Input: part model. Units: mm. Frame: model coordinates. A direction names the side the tool comes from. Coordinates: 2 decimals unless noted, no trailing zeros. Loops run counter-clockwise (first coordinate to the right, second up) from the corner with the lowest first, then second, coordinate; pieces in that order, holes last.
(1) Line query: L1, parallel to Z at x = -2.75, y = 0.9; L2, parallel to Z at x = -1.5, y = 2.5; L3, parallel to Y at x = 0.5, z = -9. Output: solid intervals per line, ascending.
(2) Contact query for flat-ended pins moving along their axis: P1, Ø4, axis at x = -2.75, z = 14, coming from the +Y side; P2, Ø1.2, axis at x = 5, y = 9, coming from the -Z side; P3, Ø2, axis at x = -3.5, z = -14.5, coming from the -Y side. Output: stop coordinate, or through.
(3) Section C-C, the plane x = -2.75. Return loops of the section in (y, z), then the cut area to 3 significant figures.
(4) Mould query, pull axis Y, two halves, no side actions, for faces 1 (the face through (1, 2, -17)), 2 (the face through (0.1, 3.1, -9.8)), 3 (the face through (0, 5, -11)). Classes: released by +Y, released by -Y, zero draft, split by the parting line, or undercut.
(5) Section B-B, the plane z = 14. Return loops of the section in (x, y).
(6) Section D-D, the plane z = 9. Return loops of the section in (x, y), then the cut area to 3 significant figures.
(7) Set-up query: faces 4 (the face through (0, 5, 11)), 5 (the face through (-1, 2, -5)), 6 (the face through (4, 8, -5)). Return all of +Z, -Z, +X, -X, +Y, -Y with unobstructed straight access to the full face (end or side cutting, diameter ignored); none if empty.
(8) Section A-A, the plane x = 0.5. Return loops of the section in (y, z), then the cut area to 3 significant figures.
Autodesk Inventor part; units mm, degrees
ref_plane "Work Plane4" through (0, 2, 0) normal (0, -1, 0) x (1, 0, 0)
ref_plane "YZ Plane" through (0, 0, 0) normal (1, 0, 0) x (0, 1, 0)
ref_plane "XZ Plane" through (0, 0, 0) normal (0, 1, 0) x (-1, 0, 0)
sketch "Sketch1" plane through (0, 0, 0) normal (0, 1, 0) x (-1, 0, 0)
  line L0 (3.75, 17) -> (-5.75, 17)
  line L1 (-5.75, 17) -> (-5.75, -17)
  line L2 (-5.75, -17) -> (3.75, -17)
  line L3 (5.75, 17) -> (-5.75, -17) construction
  line L4 (-5.75, 17) -> (5.75, -17) construction
  arc A0 (5.75, 15) -> (3.75, 17) centre (3.75, 15) ccw
  arc A1 (3.75, -17) -> (5.75, -15) centre (3.75, -15) ccw
  line L5 (-3.25, 0) -> (-3.25, 5)
  line L6 (-3.25, 0) -> (-3.25, -5)
  line L7 (-3.25, -5) -> (5.75, -5)
  line L8 (-3.25, 5) -> (5.75, 5)
  line L9 (5.75, 5) -> (5.75, 15)
  line L10 (5.75, -5) -> (5.75, -15)
  arc A2 (-0.5666, 5) -> (-0.5666, -5) centre (2.75, 0) ccw
  line L11 (-3.25, 5) -> (-5.75, 5)
  line L12 (-3.25, -5) -> (-5.75, -5)
  point P0 (2.75, 14)
  point P1 (2.75, -14)
  dimension "d0" = 11.5
  dimension "d1" = 34
  dimension "d2" = 2
  dimension "d29" = 5
  dimension "d30" = 5
  dimension "d31" = 9
  dimension "d32" = 9
  dimension "d48" = 8.5
extrude "Extrusion1" add sketch "Sketch1" along normal blind 5 contours A0 L9 L8 L11 L1 L0 | L11 L5 L6 L12 L1 | L12 L7 L10 A1 L2 L1
hole "Hole1" at (-2.75, 0, 14) at (-2.75, 0, -14) direction (0, 1, 0) diameter 3.5 depth 8
sketch "Sketch5" plane through (-5.75, 0, 5) normal (-1, 0, 0) x (0, 0, 1)
  point P0 (-5, 0)
  point P1 (4, 2.5)
  point P2 (-14, 2.5)
hole "Hole3" at (-5.75, 2.5, 9) at (-5.75, 2.5, -9) direction (1, 0, 0) diameter 2 depth 12
extrude "Extrusion4" add sketch "Sketch1" along normal blind 10.5 contours L11 L5 L6 L12 L1
ref_plane "Work Plane4" through (0, 2, 0) normal (0, -1, 0) x (1, 0, 0)
sketch "Sketch9" plane through (0, 2, 0) normal (0, -1, 0) x (1, 0, 0)
  circle A0 centre (-2.75, -14) radius 1.75
  circle A1 centre (-2.75, 14) radius 1.75
  circle A2 centre (-2.75, 14) radius 2
  circle A3 centre (-2.75, -14) radius 2
  point P0 (0, 0)
  dimension "d61" = 4
  dimension "d62" = 4
extrude "Extrusion7" cut sketch "Sketch9" along normal blind 10
properties part number "togh" material "ABS Plastic"
Report:
1. L1: z = -17 to -16, -12 to -5, 5 to 12, 16 to 17
1. L2: z = -17 to -15.22, -12.78 to -10, -8 to -5, 5 to 8, 10 to 12.78, 15.22 to 17
1. L3: y = 0 to 1.5, 3.5 to 5
2. P1: stops at y = 5
2. P2: stops at z = -5
2. P3: stops at y = 2
3. outline: (0, -17) - (5, -17) - (5, -15.75) - (2, -15.75) - (2, -16) - (0, -16) - close; (0, -12) - (2, -12) - (2, -12.25) - (5, -12.25) - (5, -5) - (0, -5) - close; (0, 5) - (5, 5) - (5, 12.25) - (2, 12.25) - (2, 12) - (0, 12) - close; (0, 16) - (2, 16) - (2, 15.75) - (5, 15.75) - (5, 17) - (0, 17) - close; hole circle Ø2 at (2.5, -9); hole circle Ø2 at (2.5, 9)
3. area: 76.7 mm2
4. face 1: zero draft
4. face 2: undercut
4. face 3: released by +Y
5. outline: (-5.75, 0) - (-4.75, 0) - (-4.75, 2) - (-4.5, 2) - (-4.5, 5) - (-5.75, 5) - close; (-1, 2) - (-0.75, 2) - (-0.75, 0) - (5.75, 0) - (5.75, 5) - (-1, 5) - close
6. outline: (-5.75, 0) - (5.75, 0) - (5.75, 1.5) - (-5.75, 1.5) - close; (-5.75, 3.5) - (5.75, 3.5) - (5.75, 5) - (-5.75, 5) - close
6. area: 34.5 mm2
7. face 4: +Z, +X, -X, +Y
7. face 5: -X, +Y, -Y
7. face 6: -Z, +X, -X, +Y
8. outline: (0, -17) - (5, -17) - (5, -5) - (0, -5) - close; (0, 5) - (5, 5) - (5, 17) - (0, 17) - close; hole circle Ø2 at (2.5, -9); hole circle Ø2 at (2.5, 9)
8. area: 114 mm2
